Work out the finished part from the listing and answer in its coordinate system (mm). Face numbers are marked on the shaded views. A direction names the side the tool comes from. Round coordinates to 2 decimals unless told otherwise and drop trailing zeros. Order: outer loops, then holes, each group sorted by start corner. A loop starts at its lowest first (then second) coordinate and runs counter-clockwise, first axis right, second up. Notation, with made-up numbers: (38.25, -33.5) - (58.25, -33.5) arc R32 cw to (58.25, -1.5) - close; hole circle Ø1 at (35, 70). An arc over 180 degrees is marked (long way). Answer in a Markdown table with one row per item.
Autodesk Inventor part; units mm, degrees
ref_plane "YZ Plane" through (0, 0, 0) normal (1, 0, 0) x (0, 1, 0)
ref_plane "XZ Plane" through (0, 0, 0) normal (0, 1, 0) x (-1, 0, 0)
ref_plane "XY Plane" through (0, 0, 0) normal (0, 0, 1) x (1, 0, 0)
sketch "スケッチ1" plane through (0, 0, 0) normal (0, 1, 0) x (-1, 0, 0)
  circle A0 centre (0, 0) radius 125
  circle A1 centre (0, 0) radius 121.5
  line L0 (118.86, 0) -> (118.86, -25.1903)
  line L1 (118.86, 0) -> (118.86, 25.1903)
  line L2 (118.86, 25.1903) -> (108.86, 25.1903)
  line L3 (108.86, 25.1903) -> (108.86, -25.1903)
  line L4 (108.86, -25.1903) -> (118.86, -25.1903)
  line L5 (118.86, -25.1903) -> (118.86, 25.1903)
  line L6 (-59.43, 102.9358) -> (-37.6146, 115.5309)
  line L7 (-59.43, 102.9358) -> (-81.2454, 90.3406)
  line L8 (-81.2454, 90.3406) -> (-76.2454, 81.6804)
  line L9 (-76.2454, 81.6804) -> (-32.6146, 106.8707)
  line L10 (-32.6146, 106.8707) -> (-37.6146, 115.5309)
  line L11 (-37.6146, 115.5309) -> (-81.2454, 90.3406)
  line L12 (-59.43, -102.9358) -> (-81.2454, -90.3406)
  line L13 (-59.43, -102.9358) -> (-37.6146, -115.5309)
  line L14 (-37.6146, -115.5309) -> (-32.6146, -106.8707)
  line L15 (-32.6146, -106.8707) -> (-76.2454, -81.6804)
  line L16 (-76.2454, -81.6804) -> (-81.2454, -90.3406)
  line L17 (-81.2454, -90.3406) -> (-37.6146, -115.5309)
  dimension "d0" = 250
  dimension "d1" = 243
  dimension "d2" = 118.86
  dimension "d3" = 10
  dimension "d6" = 360
extrude "押し出し1" add sketch "スケッチ1" along normal blind 100 contours A0 | A1 L0 L1 | L1 L0 L4 L3 L2 | L6 L7 A1 | L10 L9 L8 L7 L6 | A1 L12 L13 | L13 L12 L16 L15 L14
fillet "フィレット1" radius 8 6 edges at (37.6146, 50, -115.5309) (81.2454, 50, -90.3406) (-118.86, 50, 25.1903) (-118.86, 50, -25.1903) (81.2454, 50, 90.3406) (37.6146, 50, 115.5309)
sketch "スケッチ4" plane through (0, 100, 0) normal (0, 1, 0) x (1, 0, 0)
  line L0 (119.6242, 0) -> (119.6242, -21.2671)
  arc A0 (88.8593, -82.863) -> (88.8593, 82.863) centre (0, 0) ccw
  line L1 (119.6242, 0) -> (119.6242, 21.2671)
  arc A1 (119.6242, -21.2671) -> (119.6242, 21.2671) centre (0, 0) ccw
extrude "押し出し4" add sketch "スケッチ4" against normal blind 100
sketch "スケッチ5" plane through (119.6242, 100, -21.2671) normal (-1, 0, 0) x (0, 0, 1)
  line L0 (96.7671, -100) -> (-54.2329, -100)
  line L1 (-54.2329, -100) -> (-54.2329, -64.5)
  line L2 (-54.2329, -64.5) -> (96.7671, -64.5)
  line L3 (96.7671, -64.5) -> (96.7671, -100)
  line L4 (96.7671, -100) -> (-54.2329, -64.5) construction
  line L5 (-54.2329, -100) -> (96.7671, -64.5) construction
  line L6 (42.5342, -100) -> (0, -100)
  point P0 (21.2671, -100)
  point P1 (21.2671, -82.25)
  dimension "d20" = 151
  dimension "d21" = 35.5
  dimension "d22" = 0
extrude "押し出し5" add sketch "スケッチ5" along normal blind 30
sketch "スケッチ6" plane through (89.6242, 100, -21.2671) normal (-1, 0, 0) x (0, 0, 1)
  line L0 (96.7671, -64.5) -> (-54.2329, -64.5)
  line L1 (-54.2329, -100) -> (96.7671, -100)
  line L2 (-54.2329, -64.5) -> (96.7671, -64.5)
  line L3 (96.7671, -64.5) -> (96.7671, -100)
  line L4 (96.7671, -100) -> (-54.2329, -100)
  line L5 (-54.2329, -100) -> (-54.2329, -64.5)
  line L6 (-54.2329, -64.5) -> (-54.2329, -100)
  line L7 (-54.2329, -64.5) -> (96.7671, -64.5)
  line L8 (96.7671, -64.5) -> (96.7671, -60)
  line L9 (96.7671, -60) -> (-54.2329, -60)
  line L10 (-54.2329, -60) -> (-54.2329, -64.5)
  point P0 (21.2671, -100)
  point P1 (-54.2329, -100)
  dimension "d27" = 151
  dimension "d28" = 4.5
extrude "押し出し6" cut sketch "スケッチ6" against normal blind 100
properties part number "allwall" material "PC/ABS プラスチック"
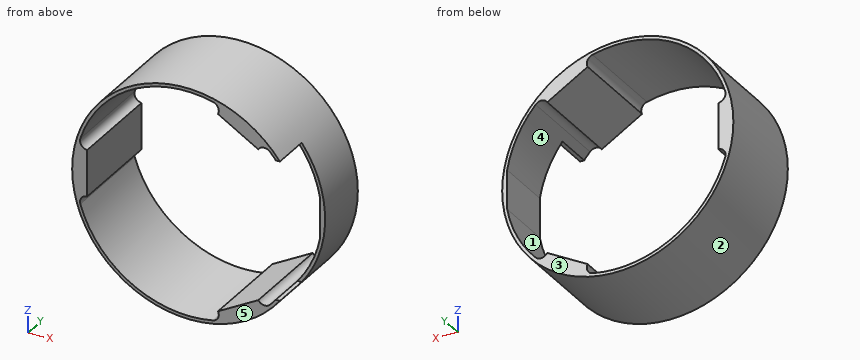
1) Find section C-C, the plane x = 0. Give the vertices of the cut face in (y, z), then the cut area to 3 significant figures.
Filled in:
| item | result |
|---|---|
| outline | (0, -125) - (100, -125) - (100, -121.5) - (0, -121.5) - close; (0, 121.5) - (100, 121.5) - (100, 125) - (0, 125) - close |
| area | 700 mm^2 |
2) The mould has two halves that part along Z. Classify the marked faces 1, 2 and 3: released by +Z, released by -Z, zero draft, split by the parting line, or undercut.
Filled in:
| item | result |
|---|---|
| face 1 | undercut |
| face 2 | split by the parting line |
| face 3 | zero draft |
3) Find section A-A, the plane y = 51.5. Give the vertices of the cut face in (x, z), then the cut area to 3 significant figures.
Filled in:
| item | result |
|---|---|
| outline | circle Ø250 at (0, 0); hole (-116.19, -35.53) arc R121.5 ccw to (27.32, -118.39) arc R8 ccw to (32.61, -106.87) - (76.25, -81.68) arc R8 ccw to (88.86, -82.86) arc R121.5 ccw to (119.62, -21.27) - (119.62, 21.27) arc R121.5 ccw to (88.86, 82.86) arc R8 ccw to (76.25, 81.68) - (32.61, 106.87) arc R8 ccw to (27.32, 118.39) arc R121.5 ccw to (-116.19, 35.53) arc R8 ccw to (-108.86, 25.2) - (-108.86, -25.2) arc R8 ccw to start |
| area | 4,690 mm^2 |
4) Which of the six approach directions +Z, -Z, +X, -X, +Y, -Y give full straight-line access (tool end or side, diameter ignored) to the marked faces 4 and 5?
Filled in:
| item | result |
|---|---|
| face 4 | +Y, -Y |
| face 5 | +Z, -Z, +X, -X, -Y |
5) Find the intervals of material crossed by probe 1 along Z at (x, y) = (-41.5, 42); probe 2 along Z at (x, y) = (-44.5, 63); probe 3 along X at (y, z) = (46, -96), in increasing order. Write a range as from..to.
Filled in:
| item | result |
|---|---|
| probe 1 | z = -117.91..-114.19, 114.19..117.91 |
| probe 2 | z = -116.81..-113.06, 113.06..116.81 |
| probe 3 | x = -80.06..-74.47, 51.44..80.06 |
6) Find section B-B, the plane z = 0. Give the vertices of the cut face in (x, y).
Filled in:
| item | result |
|---|---|
| outline | (-125, 0) - (-108.86, 0) - (-108.86, 100) - (-125, 100) - close; (119.62, 40) - (125, 40) - (125, 100) - (119.62, 100) - close |
7) Each of these flat-tipped pins is pushed along its axis until it touches: pin 1 (1.3 mm diameter, centred on x = 98.5, y = 28.5, fed in from -Z); pin 2 (6 mm diameter, centred on y = 16, z = 37.5, fed in from -X); pin 3 (1 mm diameter, centred on y = 69, z = -32, fed in from -X). Where does it stop, or does it pass through?
Filled in:
| item | result |
|---|---|
| pin 1 | stops at z = -77.78 |
| pin 2 | stops at x = -120.14 |
| pin 3 | stops at x = -120.97 |
